Geometry check sheet. Reference: the model listing, model coordinates, mm. Face numbers are marked on the shaded views. Round coordinates to 2 decimals unless told otherwise and drop trailing zeros. Use a Markdown table: item, result. Add a question column.
Item 1: Gauge pin test, flat ends, axial feed: pin 1 Ø0.6 at (x, y) = (43.5, 2) entering from +Z; pin 2 Ø2 at (x, y) = (-50.5, 2) entering from -Z; pin 3 Ø1.5 at (y, z) = (0.5, -8) entering from -X. Record the tip position at first contact, or that the pin passes through.
Item 2: Sectioned sample at A-A, the plane x = 49.5. State how many separate pieces and enclosed holes the cut face has, and give its area (3 significant figures).
Item 3: Material ranges on probe 1 along X at (y, z) = (-0.3, 0); probe 2 along Z at (x, y) = (-56, 0.3); probe 3 along X at (y, z) = (2.2, -13.5), recorded low to high. Write a range as [from, to].
Item 4: Mould release check, pull along X, two halves, no side actions. Record for the marked faces 1 and 2: pulls with the +X half, pulls with the -X half, needs draft (parallel to the pull), parting line crosses it, or undercut.
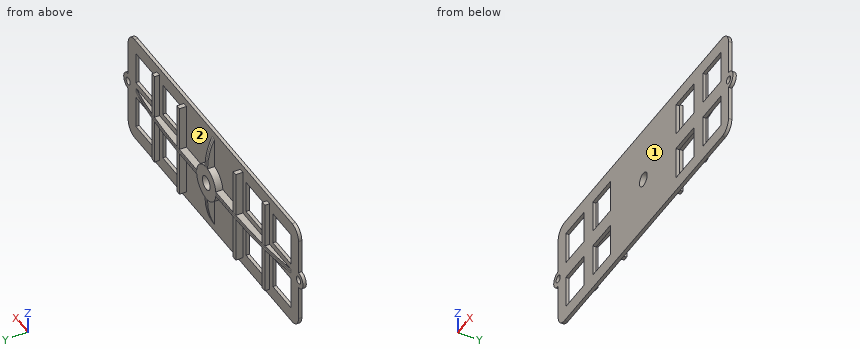
from build123d import *

# Parameters (mm, degrees)
SKETCH1_W            = 14
SKETCH1_H            = 14
BOSS_EXTRUDE1_DEPTH  = 0.7
SKETCH10_R           = 7.5
BOSS_EXTRUDE8_DEPTH  = 3
BOSS_EXTRUDE17_DEPTH = 1
SKETCH24_R           = 3
CUT_EXTRUDE5_DEPTH   = 74.970331891
SKETCH21_W           = 2
SKETCH21_H           = 3
BOSS_EXTRUDE20_DEPTH = 0.066966
BOSS_EXTRUDE22_DEPTH = 1
SKETCH26_W           = 2
SKETCH26_H           = 3
BOSS_EXTRUDE23_DEPTH = 0.066966
BOSS_EXTRUDE24_START = 1
BOSS_EXTRUDE24_DEPTH = 19.5
BOSS_EXTRUDE25_START = 1
BOSS_EXTRUDE25_DEPTH = 19.5
SKETCH30_R           = 1.6
CUT_EXTRUDE6_DEPTH   = 74.970342046
FILLET2_R            = 5


# Read off the part's stored shape, not the designer's step: Boss-Extrude24, Boss-Extrude25
with BuildPart() as part:
    # Sketch1 → Boss-Extrude1 (new, symmetric)
    with BuildSketch(Plane(origin=(0, 0, 0), x_dir=(1, 0, 0), z_dir=(0, 1, 0))):
        with BuildLine():
            Line((-66.5, 23.5), (66.5, 23.5))
            Line((66.5, 23.5), (66.5, 3.5))
            ThreePointArc((66.5, 3.5), (70, 0), (66.5, -3.5))
            Line((66.5, -3.5), (66.5, -23.5))
            Line((66.5, -23.5), (-66.5, -23.5))
            Line((-66.5, -23.5), (-66.5, -3.5))
            ThreePointArc((-66.5, -3.5), (-70, 0), (-66.5, 3.5))
            Line((-66.5, 3.5), (-66.5, 23.5))
        make_face()
        with Locations((-53.5, 10.5)):
            Rectangle(SKETCH1_W, SKETCH1_H, mode=Mode.SUBTRACT)
        with Locations((32.5, -10.5)):
            Rectangle(SKETCH1_W, SKETCH1_H, mode=Mode.SUBTRACT)
        with Locations((-53.5, -10.5)):
            Rectangle(SKETCH1_W, SKETCH1_H, mode=Mode.SUBTRACT)
        with Locations((-32.5, -10.5)):
            Rectangle(SKETCH1_W, SKETCH1_H, mode=Mode.SUBTRACT)
        with Locations((-32.5, 10.5)):
            Rectangle(SKETCH1_W, SKETCH1_H, mode=Mode.SUBTRACT)
        with Locations((53.5, -10.5)):
            Rectangle(SKETCH1_W, SKETCH1_H, mode=Mode.SUBTRACT)
        with Locations((32.5, 10.5)):
            Rectangle(SKETCH1_W, SKETCH1_H, mode=Mode.SUBTRACT)
        with Locations((53.5, 10.5)):
            Rectangle(SKETCH1_W, SKETCH1_H, mode=Mode.SUBTRACT)
    extrude(amount=BOSS_EXTRUDE1_DEPTH, both=True)

    # Sketch10 → Boss-Extrude8 (add)
    with BuildSketch(Plane(origin=(0, 0.7, 0), x_dir=(1, 0, 0), z_dir=(0, 1, 0))):
        with Locations(Location((0, 0, 0), (0, 0, 270))):
            Circle(SKETCH10_R)
    extrude(amount=BOSS_EXTRUDE8_DEPTH)

    # Sketch24 → Cut-Extrude5 (cut, through all)
    with BuildSketch(Plane(origin=(0, 3.7, 0), x_dir=(1, 0, 0), z_dir=(0, 1, 0))):
        with Locations(Location((0, 0, 0), (0, 0, 270))):
            Circle(SKETCH24_R)
    extrude(amount=-CUT_EXTRUDE5_DEPTH, mode=Mode.SUBTRACT)



with BuildPart() as body_2:
    # Sketch20 → Boss-Extrude17 (new, symmetric)
    with BuildSketch(Plane(origin=(0, 0, 0), x_dir=(0, 0, -1), z_dir=(1, 0, 0))):
        with BuildLine():
            Line((-7.5, 0.7), (-20.5, 0.7))
            add(Edge.make_bspline(
                [(-7.5, 3.7), (-14.044942682, 3.7), (-20.5, 0.7)],
                knots=[0, 0, 0, 1, 1, 1], degree=2))
            Line((-7.5, 3.7), (-7.5, 0.7))
        make_face()
    extrude(amount=BOSS_EXTRUDE17_DEPTH, both=True)


with BuildPart() as part_1:
    add(part.part)

    add(body_2.part)  # Boss-Extrude20 merges body 2
    # Sketch21 → Boss-Extrude20 (add)
    with BuildSketch(Plane(origin=(0, 0, 7.5), x_dir=(-1, 0, 0), z_dir=(0, 0, -1))):
        with Locations((0, 2.2)):
            Rectangle(SKETCH21_W, SKETCH21_H)
    extrude(amount=BOSS_EXTRUDE20_DEPTH)

    # Mirror8: part across plane


with BuildPart() as part_2:
    add(part_1.part)
    add(part_1.part.mirror(Plane.XY))



with BuildPart() as body_2_2:
    # Sketch15 → Boss-Extrude22 (new, symmetric)
    with BuildSketch(Plane.XY):
        with BuildLine():
            Line((-7.5, 0.7), (-7.5, 3.7))
            add(Edge.make_bspline(
                [(-60.5, 0.7), (-40.998326872, 3.776331264), (-27.192073984, 3.7), (-7.5, 3.7)],
                knots=[0, 0, 0, 0, 1, 1, 1, 1], degree=3))
            Line((-60.5, 0.7), (-7.5, 0.7))
        make_face()
    extrude(amount=BOSS_EXTRUDE22_DEPTH, both=True)


with BuildPart() as part_3:
    add(part_2.part)

    add(body_2_2.part)  # Boss-Extrude23 merges body 2 2
    # Sketch26 → Boss-Extrude23 (add)
    with BuildSketch(Plane(origin=(-7.5, 0, 0), x_dir=(0, 0, -1), z_dir=(1, 0, 0))):
        with Locations((0, 2.2)):
            Rectangle(SKETCH26_W, SKETCH26_H)
    extrude(amount=BOSS_EXTRUDE23_DEPTH)


with BuildPart() as body_2_3:
    # Boss-Extrude24 outline → Boss-Extrude24 (new body)
    with BuildSketch(Plane.XY.offset(BOSS_EXTRUDE24_START)):
        with BuildLine():
            Line((-42, 0.7), (-41.999999997, 2.881262224))
            add(Edge.make_bspline(
                [(-41.999999997, 2.881262224), (-42.663786895, 2.830556642), (-43.330222071, 2.776715505), (-44, 2.719545184)],
                knots=[0.657479323, 0.657479323, 0.657479323, 0.657479323, 0.696620492, 0.696620492, 0.696620492, 0.696620492], degree=3))
            Line((-44, 2.719545184), (-44, 0.7))
            Line((-44, 0.7), (-42, 0.7))
        make_face()
    extrude(amount=BOSS_EXTRUDE24_DEPTH)


with BuildPart() as body_3:
    # Mirror9: mirrored copy
    add(body_2_3.part.mirror(Plane.XY))


with BuildPart() as body_4:
    # Boss-Extrude25 outline → Boss-Extrude25 (new body)
    with BuildSketch(Plane.XY.offset(BOSS_EXTRUDE25_START)):
        with BuildLine():
            Line((-21, 0.7), (-21, 3.667005238))
            add(Edge.make_bspline(
                [(-21, 3.667005238), (-21.670951218, 3.66109998), (-22.337400803, 3.65415318), (-23.000000006, 3.645983261)],
                knots=[0.243398828, 0.243398828, 0.243398828, 0.243398828, 0.281710487, 0.281710487, 0.281710487, 0.281710487], degree=3))
            Line((-23.000000006, 3.645983261), (-23, 0.7))
            Line((-23, 0.7), (-21, 0.7))
        make_face()
    extrude(amount=BOSS_EXTRUDE25_DEPTH)


with BuildPart() as body_5:
    # Mirror10: mirrored copy
    add(body_4.part.mirror(Plane.XY))


with BuildPart() as body_6:
    # Mirror17: mirrored copy
    add(part_3.part.mirror(Plane(origin=(0, 0, 0), x_dir=(0, 0, 1), z_dir=(1, 0, 0))))


with BuildPart() as body_7:
    # Mirror17 2: mirrored copy
    add(body_4.part.mirror(Plane(origin=(0, 0, 0), x_dir=(0, 0, 1), z_dir=(1, 0, 0))))


with BuildPart() as body_8:
    # Mirror17 3: mirrored copy
    add(body_5.part.mirror(Plane(origin=(0, 0, 0), x_dir=(0, 0, 1), z_dir=(1, 0, 0))))


with BuildPart() as body_9:
    # Mirror17 4: mirrored copy
    add(body_3.part.mirror(Plane(origin=(0, 0, 0), x_dir=(0, 0, 1), z_dir=(1, 0, 0))))


with BuildPart() as body_10:
    # Mirror17 5: mirrored copy
    add(body_2_3.part.mirror(Plane(origin=(0, 0, 0), x_dir=(0, 0, 1), z_dir=(1, 0, 0))))


with BuildPart() as cut_extrude6_tool:
    # Sketch30 → Cut-Extrude6 (new, through all)
    with BuildSketch(Plane.XZ.offset(0.7)):
        with Locations(Location((-66.5, 0, 0), (0, 0, 270))):
            Circle(SKETCH30_R)
        with Locations(Location((66.5, 0, 0), (0, 0, 270))):
            Circle(SKETCH30_R)
    extrude(amount=-CUT_EXTRUDE6_DEPTH)


with BuildPart() as part_4:
    add(part_3.part)

    # Cut-Extrude6: cut by cut_extrude6_tool
    add(cut_extrude6_tool.part, mode=Mode.SUBTRACT)


with BuildPart() as body_6_1:
    add(body_6.part)

    # Cut-Extrude6: cut by cut_extrude6_tool
    add(cut_extrude6_tool.part, mode=Mode.SUBTRACT)


with BuildPart() as body_7_1:
    add(body_7.part)

    # Combine1: union body 3, body 10, body 4, part, body 2 3, body 9, body 6, body 8, body 5
    add(body_3.part)
    add(body_10.part)
    add(body_4.part)
    add(part_4.part)
    add(body_2_3.part)
    add(body_9.part)
    add(body_6_1.part)
    add(body_8.part)
    add(body_5.part)

    # Fillet2
    fillet2_edges = [body_7_1.edges().sort_by_distance(p)[0] for p in [
        (-66.5, 0, -23.5),
        (-66.5, 0, 23.5),
        (66.5, 0, 23.5),
        (66.5, 0, -23.5),
    ]]
    fillet(fillet2_edges, radius=FILLET2_R)


solid = body_7_1.part
Found:
| question | item | result |
|---|---|---|
| 1 | pin 1 | stops at z = 20.5 |
| 1 | pin 2 | stops at z = -1 |
| 1 | pin 3 | stops at x = -66.5 |
| 2 | separate pieces | 3 |
| 2 | enclosed holes | 0 |
| 2 | area | 29.6 mm2 |
| 3 | probe 1 | x = [-70, -68.1], [-64.9, -3], [3, 64.9], [68.1, 70] |
| 3 | probe 2 | z = [-23.5, -17.5], [-3.5, 3.5], [17.5, 23.5] |
| 3 | probe 3 | x = [-44, -42], [-23, -21], [-1, 1], [21, 23], [42, 44] |
| 4 | face 1 | needs draft |
| 4 | face 2 | undercut |
